Read the model definition and answer for the solid it produces. Units are mm, in the model's axes. A direction names the side the tool comes from. Give positions to 0.01 mm unless a question says otherwise; leave off trailing zeros. Order: outer loops, then holes, each group sorted by start corner. A loop starts at its lowest first (then second) coordinate and runs counter-clockwise, first axis right, second up. Notation, with made-up numbers: (14, -35.75) -> (72, -35.75) arc R24 ccw to (72, -7.75) -> close; hole circle Ø1 at (39, 11). An arc over 180 degrees is marked (long way). Use one line per item in the form item = value.
```python
from build123d import *

# Parameters (mm, degrees)
CROQUIS1_W              = 250
CROQUIS1_H              = 250
SALIENTE_EXTRUIR1_DEPTH = 20
CROQUIS2_W              = 15
CROQUIS2_H              = 30
CROQUIS2_W_2            = 30
CROQUIS2_H_2            = 15
CROQUIS2_W_3            = 40
CROQUIS2_H_3            = 40
CORTAR_EXTRUIR1_DEPTH   = 5
CROQUIS3_W              = 250
CROQUIS3_H              = 250
CROQUIS3_W_2            = 200
CROQUIS3_H_2            = 200
CORTAR_EXTRUIR2_DEPTH   = 20
CROQUIS4_W              = 200
CROQUIS4_H              = 200
SALIENTE_EXTRUIR2_DEPTH = 20
CROQUIS5_W              = 220
CROQUIS5_H              = 220
SALIENTE_EXTRUIR3_DEPTH = 40
CROQUIS6_W              = 230
CROQUIS6_H              = 230
SALIENTE_EXTRUIR4_DEPTH = 2
CORTAR_EXTRUIR5_REACH   = 176.052
CROQUIS8_R              = 9.175009618
CROQUIS8_W              = 28.599511609
CROQUIS8_H              = 46.78347923
CROQUIS8_W_2            = 46.633839802
CROQUIS8_H_2            = 27.159350596
CORTAR_EXTRUIR4_REACH   = 176.052
CROQUIS10_R             = 11.959510452


with BuildPart() as part:
    # Croquis1 → Saliente-Extruir1 (new body)
    with BuildSketch(Plane(origin=(0, 0, 0), x_dir=(1, 0, 0), z_dir=(0, 1, 0))):
        Rectangle(CROQUIS1_W, CROQUIS1_H)
    extrude(amount=SALIENTE_EXTRUIR1_DEPTH)

    # Croquis2 → Cortar-Extruir1 (cut)
    with BuildSketch(Plane(origin=(0, 20, 0), x_dir=(1, 0, 0), z_dir=(0, 1, 0))):
        with Locations((27.5, 73.5)):
            Rectangle(CROQUIS2_W, CROQUIS2_H)
        with Locations((73.5, -27.5)):
            Rectangle(CROQUIS2_W_2, CROQUIS2_H_2)
        Rectangle(CROQUIS2_W_3, CROQUIS2_H_3)
    extrude(amount=-CORTAR_EXTRUIR1_DEPTH, mode=Mode.SUBTRACT)

    # Croquis3 → Cortar-Extruir2 (cut)
    with BuildSketch(Plane(origin=(0, 20, 0), x_dir=(1, 0, 0), z_dir=(0, 1, 0))):
        Rectangle(CROQUIS3_W, CROQUIS3_H)
        Rectangle(CROQUIS3_W_2, CROQUIS3_H_2, mode=Mode.SUBTRACT)
    extrude(amount=-CORTAR_EXTRUIR2_DEPTH, mode=Mode.SUBTRACT)

    # Croquis4 → Saliente-Extruir2 (add)
    with BuildSketch(Plane.XZ):
        Polygon((115, -96.500184321), (115, -115), (-115, -115), (-115, -98.664064905), (-115, 115), (-100, 115), (115, 115), (115, 96.335935095), align=None)
        Rectangle(CROQUIS4_W, CROQUIS4_H, mode=Mode.SUBTRACT)
    extrude(amount=-SALIENTE_EXTRUIR2_DEPTH)

    # Croquis5 → Saliente-Extruir3 (add)
    with BuildSketch(Plane(origin=(0, 20, 0), x_dir=(1, 0, 0), z_dir=(0, 1, 0))):
        Polygon((115, 115), (-115, 115), (-115, 110.241153541), (-115, -107.327290452), (-115, -115), (-108.298578148, -115), (115, -115), (115, -107.327290452), (115, 110.241153541), align=None)
        Rectangle(CROQUIS5_W, CROQUIS5_H, mode=Mode.SUBTRACT)
    extrude(amount=SALIENTE_EXTRUIR3_DEPTH)

    # Croquis6 → Saliente-Extruir4 (add)
    with BuildSketch(Plane(origin=(0, 60, 0), x_dir=(1, 0, 0), z_dir=(0, 1, 0))):
        Rectangle(CROQUIS6_W, CROQUIS6_H)
    extrude(amount=SALIENTE_EXTRUIR4_DEPTH)

    # Croquis8 → Cortar-Extruir5 (cut, up to next)
    with BuildSketch(Plane(origin=(0, 62, 0), x_dir=(1, 0, 0), z_dir=(0, 1, 0)), mode=Mode.PRIVATE) as cortar_extruir5_sk1:
        with Locations(Location((0, 0, 0), (0, 0, 270))):
            Circle(CROQUIS8_R)
    cortar_extruir5_tool1 = extrude(cortar_extruir5_sk1.sketch, amount=-CORTAR_EXTRUIR5_REACH, mode=Mode.PRIVATE) & part.part
    # Croquis8 → Cortar-Extruir5 (cut, up to next)
    with BuildSketch(Plane(origin=(0, 62, 0), x_dir=(1, 0, 0), z_dir=(0, 1, 0)), mode=Mode.PRIVATE) as cortar_extruir5_sk2:
        with Locations((53.986056935, 0)):
            Rectangle(CROQUIS8_W, CROQUIS8_H)
    cortar_extruir5_tool2 = extrude(cortar_extruir5_sk2.sketch, amount=-CORTAR_EXTRUIR5_REACH, mode=Mode.PRIVATE) & part.part
    # Croquis8 → Cortar-Extruir5 (cut, up to next)
    with BuildSketch(Plane(origin=(0, 62, 0), x_dir=(1, 0, 0), z_dir=(0, 1, 0)), mode=Mode.PRIVATE) as cortar_extruir5_sk3:
        with Locations((0, 53.729056372)):
            Rectangle(CROQUIS8_W_2, CROQUIS8_H_2)
    cortar_extruir5_tool3 = extrude(cortar_extruir5_sk3.sketch, amount=-CORTAR_EXTRUIR5_REACH, mode=Mode.PRIVATE) & part.part
    add(cortar_extruir5_tool1.solids().sort_by_distance((0, 62, 0))[0], mode=Mode.SUBTRACT)
    add(cortar_extruir5_tool2.solids().sort_by_distance((53.986057, 62, 0))[0], mode=Mode.SUBTRACT)
    add(cortar_extruir5_tool3.solids().sort_by_distance((0, 62, -53.729056))[0], mode=Mode.SUBTRACT)

    # Croquis10 → Cortar-Extruir4 (cut, up to next)
    with BuildSketch(Plane(origin=(0, 62, 0), x_dir=(1, 0, 0), z_dir=(0, 1, 0)), mode=Mode.PRIVATE) as cortar_extruir4_sk1:
        with Locations(Location((0, 0, 0), (0, 0, 270))):
            Circle(CROQUIS10_R)
    cortar_extruir4_tool1 = extrude(cortar_extruir4_sk1.sketch, amount=-CORTAR_EXTRUIR4_REACH, mode=Mode.PRIVATE) & part.part
    add(cortar_extruir4_tool1.solids().sort_by_distance((0, 62, 0))[0], mode=Mode.SUBTRACT)


solid = part.part
```
Item 1: The part is cut by section C-C on y = 23. Give the vertices of the cut face in (x, z).
Checks:
outline = (-115, -115) -> (115, -115) -> (115, 115) -> (-115, 115) -> close; hole (-110, -110) -> (110, -110) -> (110, 110) -> (-110, 110) -> close
Item 2: The part is cut by section B-B on x = 0. Give the vertices of the cut face in (y, z), and give its area (3 significant figures).
Checks:
outline = (0, -115) -> (62, -115) -> (62, -67.31) -> (60, -67.31) -> (60, -110) -> (20, -110) -> (20, -20) -> (15, -20) -> (15, 20) -> (20, 20) -> (20, 110) -> (60, 110) -> (60, 11.96) -> (62, 11.96) -> (62, 115) -> (0, 115) -> close; (60, -40.15) -> (62, -40.15) -> (62, -11.96) -> (60, -11.96) -> close
area = 5,160 mm²
Item 3: Straight lines are drawn through the part: L1, parallel to X at y = 60.5, z = 0; L2, parallel to X at y = 42, z = 8; L3, parallel to Y at x = -35, z = -100. For each, find the intervals that lie inside material, in ascending order. Write a range as from..to.
Checks:
L1 = -115..-11.96, 11.96..39.69, 68.29..115
L2 = -115..-110, 110..115
L3 = 0..20, 60..62
Item 4: The part is cut by section D-D on x = -89.5. Give the vertices of the cut face in (y, z).
Checks:
outline = (0, -115) -> (62, -115) -> (62, 115) -> (0, 115) -> close; hole (20, -110) -> (60, -110) -> (60, 110) -> (20, 110) -> close
Item 5: Which of the six approach directions +Z, -Z, +X, -X, +Y, -Y give full straight-line access (tool end or side, diameter ignored) to faces 1 (the flat face through (-110, 40, 2)), 2 (the flat face through (-2, 62, 24)), 3 (the cylindrical face through (11.858, 61.014, -1.557))?
Checks:
face_1 = none
face_2 = +Z, -Z, +X, -X, +Y
face_3 = +Y
Item 6: The part is cut by section A-A on z = 0. Give the vertices of the cut face in (x, y).
Checks:
outline = (-115, 0) -> (115, 0) -> (115, 62) -> (68.29, 62) -> (68.29, 60) -> (110, 60) -> (110, 20) -> (20, 20) -> (20, 15) -> (-20, 15) -> (-20, 20) -> (-110, 20) -> (-110, 60) -> (-11.96, 60) -> (-11.96, 62) -> (-115, 62) -> close; (11.96, 60) -> (39.69, 60) -> (39.69, 62) -> (11.96, 62) -> close
Item 7: Determine the mould class of faces 4 (the flat face through (35, 18, -73)), 5 (the flat face through (115, 31, 2)) for opening direction Z: +Z half, -Z half, draft (parallel to the pull), parting line (faces both ways), or undercut.
Checks:
face_4 = undercut
face_5 = draft
Item 8: Given pin 1 Ø12 at (x, z) = (-3, -1.5) entering from +Y, flat-ended and moving along its own axis, determine where the tip first touches the part or whether it passes through.
Checks:
pin_1 = 15
